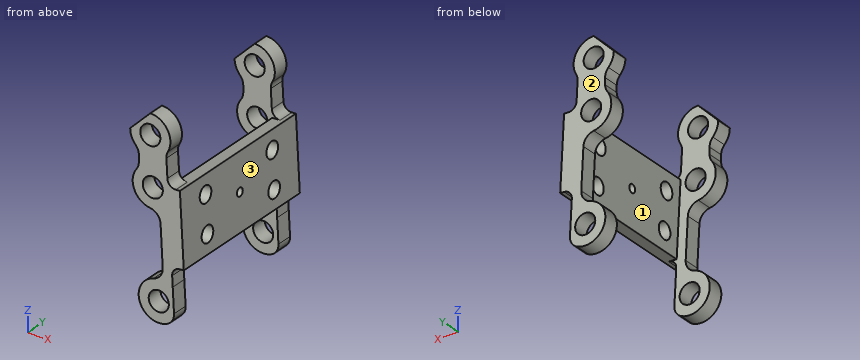
from build123d import *

# Parameters (mm, degrees)
SKETCH2_R           = 2.5
BOSS_EXTRUDE3_DEPTH = 4
BOSS_EXTRUDE4_DEPTH = 40
FILLET1_R           = 2
SKETCH4_R           = 2
SKETCH4_R_2         = 1
CUT_EXTRUDE1_DEPTH  = 10
FILLET3_R           = 3
FILLET4_R           = 3


with BuildPart() as part:
    # Sketch2 → Boss-Extrude3 (new body)
    with BuildSketch(Plane(origin=(0, 0, 0), x_dir=(1, 0, 0), z_dir=(0, 1, 0))):
        with BuildLine():
            ThreePointArc((83.62627208, 73.409646321), (82.043328915, 71.619198109), (81.472187529, 69.298592288))
            Line((81.472187529, 69.298592288), (86.472187529, 64.298592288))
            ThreePointArc((86.472187529, 64.298592288), (90.961711336, 67.097643404), (90.424672494, 72.360921892))
            Line((90.424672494, 72.360921892), (90.926689774, 81.686644374))
            Line((90.926689774, 81.686644374), (92.048119667, 102.518883374))
            Line((92.048119667, 102.518883374), (92.450855554, 110.000305351))
            ThreePointArc((92.450855554, 110.000305351), (83.843337657, 108.444197301), (89.726552777, 101.971283238))
            Line((89.726552777, 101.971283238), (88.863578179, 85.80252536))
            ThreePointArc((88.863578179, 85.80252536), (82.866493913, 83.799788509), (83.62627208, 77.522949199))
            Line((83.62627208, 77.522949199), (83.62627208, 73.409646321))
        make_face()
        with Locations(Location((86.472187529, 69.298592288, 0), (0, 0, 270))):
            Circle(SKETCH2_R, mode=Mode.SUBTRACT)
        with Locations(Location((87.092070964, 81.126869023, 0), (0, 0, 270))):
            Circle(SKETCH2_R, mode=Mode.SUBTRACT)
        with Locations(Location((88.578200606, 106.837625529, 0), (0, 0, 270))):
            Circle(SKETCH2_R, mode=Mode.SUBTRACT)
    boss_extrude3 = extrude(amount=BOSS_EXTRUDE3_DEPTH)

    # Sketch3 → Boss-Extrude4 (add)
    with BuildSketch(Plane(origin=(0, 4, 0), x_dir=(1, 0, 0), z_dir=(0, 1, 0))):
        Polygon((91.800965367, 97.92762227), (90.833399946, 79.953646162), (93.833399946, 79.792151774), (94.800965367, 97.766127883), align=None)
    extrude(amount=-BOSS_EXTRUDE4_DEPTH)

    # Mirror1: Boss-Extrude3 across plane
    add(boss_extrude3.mirror(Plane.ZX.offset(-16)))

    # Fillet1
    fillet1_edges = [part.edges().sort_by_distance(p)[0] for p in [
        (90.833399946, -34, -79.953646162),
        (91.800965367, -34, -97.92762227),
        (91.800965367, 2, -97.92762227),
        (90.833399946, 2, -79.953646162),
    ]]
    fillet(fillet1_edges, radius=FILLET1_R)

    # Sketch4 → Cut-Extrude1 (cut)
    with BuildSketch(Plane(origin=(86.279355648, 0, 4.6445439), x_dir=(-0.05375363451621944, 0, 0.9985542282601866), z_dir=(-0.9985542282601865, 0, -0.05375363451621943))):
        with Locations((-89.220676822, -4.5)):
            Circle(SKETCH4_R)
        with Locations(Location((-98.220676822, -4.5, 0), (0, 0, 180))):
            Circle(SKETCH4_R)
        with Locations(Location((-89.220676822, -27.5, 0), (0, 0, 180))):
            Circle(SKETCH4_R)
        with Locations((-98.220676822, -27.5)):
            Circle(SKETCH4_R)
        with Locations((-93.720676822, -16)):
            Circle(SKETCH4_R_2)
    extrude(amount=-CUT_EXTRUDE1_DEPTH, mode=Mode.SUBTRACT)

    # Fillet3
    fillet3_edges = [part.edges().sort_by_distance(p)[0] for p in [
        (92.450855554, 2, -110.000305351),
        (90.424672494, 2, -72.360921892),
        (83.62627208, 2, -73.409646321),
        (83.62627208, 2, -77.522949199),
        (89.726552777, 2, -101.971283238),
        (92.450855554, -34, -110.000305351),
        (89.726552777, -34, -101.971283238),
        (90.424672494, -34, -72.360921892),
        (83.62627208, -34, -73.409646321),
        (83.62627208, -34, -77.522949199),
    ]]
    fillet(fillet3_edges, radius=FILLET3_R)

    # Fillet4
    fillet4_edges = [part.edges().sort_by_distance(p)[0] for p in [
        (88.863578179, 2, -85.80252536),
        (88.863578179, -34, -85.80252536),
    ]]
    fillet(fillet4_edges, radius=FILLET4_R)


solid = part.part
Work out the finished part from the listing and answer in its coordinate system (mm). Face numbers are marked on the shaded views. Coordinates: 2 decimals unless noted, no trailing zeros. Loops run counter-clockwise (first coordinate to the right, second up) from the corner with the lowest first, then second, coordinate; pieces in that order, holes last. Notation, with made-up numbers: (-31.5, 66) -> (0.5, 66) arc R28 ccw to (0.5, 100) -> close; hole circle Ø7 at (16, 23). An arc over 180 degrees is marked (long way). Answer as CSV lines item,"result".
1) The part is cut by section C-C (z = -77). Give the vertices of the cut face in (x, y), and give its area (3 significant figures).
A:
outline,"(83.57, -36) -> (90.67, -36) -> (90.67, -32) -> (83.57, -32) -> close; (83.57, 0) -> (90.67, 0) -> (90.67, 4) -> (83.57, 4) -> close"
area,"56.8 mm²"
2) The part is cut by section A-A (y = -33). Give the vertices of the cut face in (x, z) (1 decimal).
A:
outline,"(81.5, -69.3) arc R5 ccw to (82.8, -72.7) arc R3 cw to (83.6, -74.8) -> (83.6, -76.4) arc R3 cw to (83.1, -78.2) arc R5 ccw to (86.4, -86.1) arc R3 cw to (89, -88.9) -> (89.6, -98.9) arc R3 cw to (87.3, -102) arc R5 ccw (long way) to (90.6, -111.4) arc R3 ccw to (92.4, -108.5) -> (91.9, -99.9) arc R2 cw to (93.8, -97.8) -> (94.8, -97.8) -> (93.8, -79.8) -> (92.8, -79.8) arc R2 cw to (90.7, -78) -> (90.5, -73.3) arc R3 cw to (90.8, -71.7) arc R5 ccw to (86.5, -64.3) -> close; hole circle Ø5 at (86.5, -69.3); hole circle Ø5 at (87.1, -81.1); hole circle Ø5 at (88.6, -106.8)"
3) Flat-ended cylindrical pins translate along their axes: pin 1 (5 mm diameter, centred on x = 88.5, y = -29, fed in from +Z); pin 2 (6 mm diameter, centred on x = 85, z = -97.5, fed in from +Y); pin 3 (1.3 mm diameter, centred on y = 2.5, z = -75.5, fed in from -X); pin 4 (4 mm diameter, centred on y = -4, z = -93, fed in from +X). Find the tip coordinate at first contact, or state that the pin passes through.
A:
pin 1,"stops at z = -79.94"
pin 2,"passes through"
pin 3,"stops at x = 83.63"
pin 4,"stops at x = 94.65"
4) Straight lines are drawn through the part: probe 1 along Y at (x, z) = (90, -94); probe 2 along Z at (x, y) = (93, -27); probe 3 along Z at (x, y) = (90, -33.5). For each, find the intervals that lie inside material, in ascending order.
A:
probe 1,"y = -36 to -32, 0 to 4"
probe 2,"z = -97.86 to -95.3, -91.42 to -86.28, -82.4 to -79.84"
probe 3,"z = -111.63 to -108.89, -104.78 to -65.76"
5) For a pull along Y with two mould halves and no side action, classify the marked faces 1, 2 and 3 as released by +Y, released by -Y, zero draft, split by the parting line, or undercut.
A:
face 1,"undercut"
face 2,"released by +Y"
face 3,"zero draft"
6) The part is cut by section D-D (z = -96.5). Give the vertices of the cut face in (x, y), and give its area (3 significant figures).
A:
outline,"(89.43, -36) -> (94.73, -36) -> (94.73, 4) -> (89.43, 4) -> (89.43, 0) -> (91.72, 0) -> (91.72, -32) -> (89.43, -32) -> close"
area,"139 mm²"
7) The part is cut by section B-B (y = -5.5). Give the vertices of the cut face in (x, z).
A:
outline,"(90.83, -79.95) -> (90.98, -82.72) -> (93.98, -82.56) -> (93.83, -79.79) -> close; (91.17, -86.18) -> (91.47, -91.7) -> (94.47, -91.54) -> (94.17, -86.02) -> close; (91.65, -95.16) -> (91.8, -97.93) -> (94.8, -97.77) -> (94.65, -95) -> close"
